from build123d import *

# Parameters (mm, degrees)
F0_R     = 34.29
F0_R_2   = 27.94
F1_DEPTH = 38.1
F3_DEPTH = 38.1
F4_R     = 6.35
F5_R     = 5.08
F6_R     = 5.08


with BuildPart() as f1:
    # F0 (on Front) → F1 (new body)
    with BuildSketch(Plane.XZ):
        Circle(F0_R)
        Circle(F0_R_2, mode=Mode.SUBTRACT)
    extrude(amount=-F1_DEPTH)

    # F2 (on face) → F3 (join)
    with BuildSketch(Plane.XZ):
        with BuildLine():
            ThreePointArc((18.723981822, -28.7265835896), (-0.3921055503, -34.2877580667), (-19.376018178, -28.2908822691))
            Line((-19.376018178, -28.2908822691), (-19.376018178, -159.8299160348))
            Line((-19.376018178, -159.8299160348), (18.723981822, -160.462572118))
            Line((18.723981822, -160.462572118), (18.723981822, -28.7265835896))
        make_face()
    extrude(amount=-F3_DEPTH)

    # F4
    f4_edges = [f1.edges().sort_by_distance(p)[0] for p in [
        (-0.326018, 0, -160.146244),
        (-0.326018, 38.1, -160.146244),
        (18.723982, 19.05, -160.462572),
        (-19.376018, 19.05, -159.829916),
    ]]
    fillet(f4_edges, radius=F4_R)

    # F5
    f5_edges = [f1.edges().sort_by_distance(p)[0] for p in [
        (-27.94, 0, 0),
    ]]
    fillet(f5_edges, radius=F5_R)

    # F6
    f6_edges = [f1.edges().sort_by_distance(p)[0] for p in [
        (-27.94, 38.1, 0),
    ]]
    fillet(f6_edges, radius=F6_R)


solid = f1.part
Geometry: final body of the model. Coordinates: model frame, mm. A direction names the side the tool comes from. Give positions to 0.01 mm unless a question says otherwise; leave off trailing zeros. Write each loop counter-clockwise with the first axis right and the second up, starting at its lowest first coordinate (ties: lowest second). Pieces come first, ordered by that corner, then holes. Notation, with made-up numbers: (-25, -2) - (-13, -2) arc R19 ccw to (-13, 9) - close; hole circle Ø3 at (64, -22.75). An arc over 180 degrees is marked (long way). Return JSON: item names as keys, results as strings. Group by question number.
1) First-contact query: P1, Ø11.5, axis at y = 20.5, z = -121.5, coming from the -X side; P2, Ø1.5, axis at y = 14, z = -27, coming from the -X side; P3, Ø1, axis at y = 34, z = -24.5, coming from the +X side. Flat tips, straight axial feed; report the tip coordinate or a pass-through.
2) Section A-A on y = 16.5. Return the cut outline in (x, z), plus the area to 3 significant figures.
3) Line query: line 1 (X direction, y = 3, z = -77); line 2 (Z direction, x = 0, y = 22.25); line 3 (Z direction, x = 2, y = 5.5). Output: solid intervals per line, ascending.
4) Mould query, pull axis Z, two halves, no side actions, for faces 5 (the cylindrical face through (16.78, 19.32, -158.58)), 6 (the cylindrical face through (-3.64, 18.85, 27.7)), 7 (the cylindrical face through (1.62, 18.78, 34.25)), 8 (the flat face through (0, 38.1, -80)). Classes: released by +Z, released by -Z, zero draft, split by the parting line, or undercut.
5) Set-up query: faces 1 (the cylindrical face through (-0.14, 36.19, -158.34)), 2 (the flat face through (18.724, 19, -92)), 3 (the cylindrical face through (-0.14, 1.91, -158.34)), 4 (the flat face through (-19.376, 19, -90)). Return all of +Z, -Z, +X, -X, +Y, -Y with unobstructed straight access to the full face (end or side cutting, diameter ignored); none if empty.
6) Section C-C on z = -118. Return the cut outline in (x, y).
7) Section D-D on y = 35.5. Return the cut outline in (x, z), plus the area to 3 significant figures.
8) Section B-B on z = 0. Return the cut outline in (x, y), plus the area to 3 significant figures.
Filled in:
{
 "1": {"P1": "stops at x = -19.38", "P2": "stops at x = -22.06", "P3": "stops at x = 24.49"},
 "2": {"outline": "(-19.38, -153.58) arc R6.35 ccw to (-13.13, -159.93) - (12.27, -160.36) arc R6.35 ccw to (18.72, -154.01) - (18.72, -28.73) arc R34.29 ccw (long way) to (-19.38, -28.29) - close; hole circle Ø55.88 at (0, 0)", "area": "6,090 mm^2"},
 "3": {"line 1": "x = -19.38 to 18.72", "line 2": "z = -160.15 to -27.94, 27.94 to 34.29", "line 3": "z = -160.13 to -27.87, 27.87 to 34.23"},
 "4": {"face 5": "released by -Z", "face 6": "undercut", "face 7": "split by the parting line", "face 8": "zero draft"},
 "5": {"face 1": "-Z, -X, +Y", "face 2": "-Z, +X, +Y, -Y", "face 3": "-Z, -X, -Y", "face 4": "-Z, -X, +Y, -Y"},
 "6": {"outline": "(-19.38, 0) - (18.72, 0) - (18.72, 38.1) - (-19.38, 38.1) - close"},
 "7": {"outline": "(-19.38, -153.58) arc R6.35 ccw to (-16.86, -158.65) - (16.04, -159.19) arc R6.35 ccw to (18.72, -154.01) - (18.72, -28.73) arc R34.29 ccw (long way) to (-19.38, -28.29) - close; hole circle Ø57.17 at (0, 0)", "area": "5,940 mm^2"},
 "8": {"outline": "(-34.29, 0) - (-33.02, 0) arc R5.08 ccw to (-27.94, 5.08) - (-27.94, 33.02) arc R5.08 ccw to (-33.02, 38.1) - (-34.29, 38.1) - close; (27.94, 5.08) arc R5.08 ccw to (33.02, 0) - (34.29, 0) - (34.29, 38.1) - (33.02, 38.1) arc R5.08 ccw to (27.94, 33.02) - close", "area": "462 mm^2"}
}
